The model under review builds one solid part; all positions refer to its coordinate system, in mm. Coordinates: 2 decimals unless noted, no trailing zeros. Write each loop counter-clockwise with the first axis right and the second up, starting at its lowest first coordinate (ties: lowest second). Pieces come first, ordered by that corner, then holes. Notation, with made-up numbers: (3.25, 64) - (38.25, 64) arc R14 ccw to (38.25, 81) - close; hole circle Ø6 at (27, 87). An arc over 180 degrees is marked (long way). Put each result on its own line as item: value. Start each with the question number.
Item 1: Consider section C-C on y = 30. Give the boundary of the cut face in (x, z) (3 decimals), then the cut area to 3 significant figures.
Item 2: Consider section B-B on z = 6. Give the boundary of the cut face in (x, y).
Item 3: Mouldability with a two-part tool opening along X and no side actions: class faces 1 (the face through (-20, 39, 0)), 2 (the face through (0.28, 44.874, 13.053)), 3 (the face through (-11.715, 25.26, -2.601)) as pulls with the +X half, pulls with the -X half, needs draft (parallel to the pull), parting line crosses it, or undercut.
Item 4: Consider section D-D on z = 17. Give the boundary of the cut face in (x, y), then the cut area to 3 significant figures.
Item 5: Consider section A-A on x = -5.5. Give the boundary of the cut face in (y, z), then the cut area to 3 significant figures.
Item 6: To check wall thickness, follow L1, parallel to Z at x = 0, y = 18; L2, parallel to X at y = 48.5, z = 0; L3, parallel to Z at x = -5, y = 40. State the ranges of each line that lie inside material, in increasing order. Write a range as [from, to].
Item 7: For pin 1 (8 mm diameter, centred on y = 24.5, z = 7, fed in from +X); pin 2 (2 mm diameter, centred on y = 46.5, z = -9, fed in from +X), all flat-tipped, find the tip position at first contact; note any pin that passes through.
```python
from build123d import *

# Parameters (mm, degrees)
SKETCH_1_W               = 40
SKETCH_1_H               = 40
SKETCH_1_R               = 12
EXTRUDE_1_DEPTH          = 80
CUT_EXTRUDE_2_DEPTH      = 85.852813742
CUT_EXTRUDE_2_DEPTH_BACK = 85.852813742


with BuildPart() as part:
    # 草圖1 → 填料-伸長1 (new body)
    with BuildSketch(Plane(origin=(0, 0, 0), x_dir=(1, 0, 0), z_dir=(0, 1, 0))):
        Rectangle(SKETCH_1_W, SKETCH_1_H)
        with Locations(Location((0, 0, 0), (0, 0, 270))):
            Circle(SKETCH_1_R, mode=Mode.SUBTRACT)
    extrude(amount=EXTRUDE_1_DEPTH)

    # 草圖2 → 除料-伸長2 (cut, two sides: drawn at the far end of the back side and taken through both)
    with BuildSketch(Plane.XY.offset(-CUT_EXTRUDE_2_DEPTH_BACK)):
        Polygon((114.4427191, -152.861620189), (20, 10.717967697), (-20, 80), (-114.4427191, 243.579587886), (212.716456672, 432.465026086), (441.601894872, 36.023818011), align=None)
    extrude(amount=CUT_EXTRUDE_2_DEPTH + CUT_EXTRUDE_2_DEPTH_BACK, mode=Mode.SUBTRACT)


solid = part.part
```
Report:
1. outline: (-20, -20) - (8.868, -20) - (8.868, -8.085) arc R12 cw (long way) to (8.868, 8.085) - (8.868, 20) - (-20, 20) - close
1. area: 737 mm²
2. outline: (-20, 0) - (-10.39, 0) - (-10.39, 63.36) - (-20, 80) - close; (10.39, 0) - (20, 0) - (20, 10.72) - (10.39, 27.36) - close
3. face 1: pulls with the -X half
3. face 2: pulls with the +X half
3. face 3: undercut
4. outline: (-20, 0) - (20, 0) - (20, 10.72) - (-20, 80) - close
4. area: 1,810 mm²
5. outline: (0, -20) - (54.89, -20) - (54.89, -10.67) - (0, -10.67) - close; (0, 10.67) - (54.89, 10.67) - (54.89, 20) - (0, 20) - close
5. area: 1,020 mm²
6. L1: [-20, -12], [12, 20]
6. L2: [-20, -12]
6. L3: [-20, -10.91], [10.91, 20]
7. pin 1: x = 14.35
7. pin 2: x = -6.63
